Design review of the part built by this model. Coordinates are the model's own, in mm. A direction names the side the tool comes from. Give positions to 0.01 mm unless a question says otherwise; leave off trailing zeros. Order: outer loops, then holes, each group sorted by start corner. A loop starts at its lowest first (then second) coordinate and runs counter-clockwise, first axis right, second up. Notation, with made-up numbers: (-16, 41.25) -> (34, 41.25) arc R23 ccw to (34, 77.25) -> close; hole circle Ø6 at (-23, 35). An arc over 180 degrees is marked (long way). Use a Markdown table: item, result. Add a question column.
```python
from build123d import *

# Parameters (mm, degrees)
F0_W     = 100
F0_H     = 100
F1_DEPTH = 5
F2_W     = 100
F2_H     = 100
F2_W_2   = 90
F2_H_2   = 90
F3_DEPTH = 50


with BuildPart() as f1:
    # F0 (on Top) → F1 (new body)
    with BuildSketch(Plane.XY):
        with Locations((0, 0.521898)):
            Rectangle(F0_W, F0_H)
    extrude(amount=-F1_DEPTH)

    # F2 (on face) → F3 (join)
    with BuildSketch(Plane.XY):
        with Locations((0, 0.521898)):
            Rectangle(F2_W, F2_H)
        with Locations((0, 0.521898)):
            Rectangle(F2_W_2, F2_H_2, mode=Mode.SUBTRACT)
    extrude(amount=F3_DEPTH)


solid = f1.part
```
1) The part is to be moulded in two halves that separate along Y. For faces 3 (the flat face through (-1, -49.478, 22)), 4 (the flat face through (50, 0, 22)), 5 (the flat face through (-1, 50.522, 22)), 6 (the flat face through (-1, 45.522, 25)), say which applies: +Y half, -Y half, draft (parallel to the pull), parting line (faces both ways), or undercut.
2) Add section A-A (z = 7.5). Give the boundary of the cut face in (x, y), then the cut area to 3 significant figures.
3) Add section B-B (y = -10.5). Give the boundary of the cut face in (x, z).
4) For L1, parallel to X at y = 27.5, z = 13; L2, parallel to Y at x = -23, z = 26; L3, parallel to Z at x = 26, y = 42, list the stretches that pass through material, from the lowest coordinate up. Write a range as [from, to].
5) Machinability: for faces 1 (the flat face through (-45, 0, 25)), 2 (the flat face through (-1, 1, -5)), which of the approach directions +Z, -Z, +X, -X, +Y, -Y give a long, thin tool a straight path to every point of the face, cutting with its end or side? Answer none if there is none.
6) Add section C-C (x = 36). Give the boundary of the cut face in (y, z), then the cut area to 3 significant figures.
7) Insertion check: pin 1 (12 mm diameter, centred on x = -26, y = 28, fed in from +Z). The pin has a flat end and moves straight along its axis. Give the tip position at first contact, or say it passes through.
Worked answers:
| question | item | result |
|---|---|---|
| 1 | face 3 | -Y half |
| 1 | face 4 | draft |
| 1 | face 5 | +Y half |
| 1 | face 6 | undercut |
| 2 | outline | (-50, -49.48) -> (50, -49.48) -> (50, 50.52) -> (-50, 50.52) -> close; hole (-45, -44.48) -> (45, -44.48) -> (45, 45.52) -> (-45, 45.52) -> close |
| 2 | area | 1,900 mm^2 |
| 3 | outline | (-50, -5) -> (50, -5) -> (50, 50) -> (45, 50) -> (45, 0) -> (-45, 0) -> (-45, 50) -> (-50, 50) -> close |
| 4 | L1 | [-50, -45], [45, 50] |
| 4 | L2 | [-49.48, -44.48], [45.52, 50.52] |
| 4 | L3 | [-5, 0] |
| 5 | face 1 | +Z |
| 5 | face 2 | -Z, +X, -X, +Y, -Y |
| 6 | outline | (-49.48, -5) -> (50.52, -5) -> (50.52, 50) -> (45.52, 50) -> (45.52, 0) -> (-44.48, 0) -> (-44.48, 50) -> (-49.48, 50) -> close |
| 6 | area | 1,000 mm^2 |
| 7 | pin 1 | z = 0 |
